```python
from build123d import *

# Parameters (mm, degrees)
F0_W     = 203.2
F0_H     = 254
F0_R     = 25.4
F1_DEPTH = 50.8
F2_R     = 5.08


with BuildPart() as f1:
    # F0 (on Top) → F1 (new body)
    with BuildSketch(Plane.XY):
        with Locations((101.6, 127)):
            Rectangle(F0_W, F0_H)
        with Locations((101.6, 50.8)):
            Circle(F0_R, mode=Mode.SUBTRACT)
        with Locations((101.6, 203.2)):
            Circle(F0_R, mode=Mode.SUBTRACT)
    extrude(amount=F1_DEPTH)

    # F2
    f2_edges = [f1.edges().sort_by_distance(p)[0] for p in [
        (101.6, 254, 0),
        (76.2, 203.2, 0),
        (0, 127, 0),
        (0, 127, 50.8),
        (0, 254, 25.4),
        (76.2, 50.8, 0),
        (203.2, 127, 0),
        (101.6, 0, 0),
        (0, 0, 25.4),
        (76.2, 203.2, 50.8),
        (76.2, 50.8, 50.8),
        (203.2, 0, 25.4),
        (101.6, 0, 50.8),
        (203.2, 127, 50.8),
    ]]
    fillet(f2_edges, radius=F2_R)


solid = f1.part
```
Read the model definition and answer for the solid it produces. Units are mm, in the model's axes. Round coordinates to 2 decimals unless told otherwise and drop trailing zeros. Loops run counter-clockwise (first coordinate to the right, second up) from the corner with the lowest first, then second, coordinate; pieces in that order, holes last. Notation, with made-up numbers: (-4, -37) -> (39, -37) arc R26 cw to (39, -2) -> close; hole circle Ø3 at (27.25, 7.25). An arc over 180 degrees is marked (long way). One line per item, written item: value.
1) The mould has two halves that part along Y. Classify faces 1 (the face through (98.293, 228.384, 25.116)), 2 (the face through (102.951, 1.449, 49.272)), 3 (the face through (201.751, 131.282, 1.528)): pulls with the +Y half, pulls with the -Y half, needs draft (parallel to the pull), parting line crosses it, or undercut.
Answer list:
face 1: undercut
face 2: pulls with the -Y half
face 3: needs draft
2) Consider L1, parallel to Y at x = 101, z = 25; L2, parallel to X at y = 203, z = 26; L3, parallel to Y at x = 103.5, z = 44.5. Determine where each line is inside the solid, lowest interval first. Write a range as [from, to].
Answer list:
L1: y = [0, 25.41], [76.19, 177.81], [228.59, 254]
L2: x = [0, 76.2], [127, 203.2]
L3: y = [0, 25.47], [76.13, 177.87], [228.53, 254]
3) A cutting plane is placed at A-A (x = 101.6). Determine the outline of the cut face in (y, z), and give its area (3 significant figures).
Answer list:
outline: (0, 5.08) arc R5.08 ccw to (5.08, 0) -> (20.32, 0) arc R5.08 ccw to (25.4, 5.08) -> (25.4, 45.72) arc R5.08 ccw to (20.32, 50.8) -> (5.08, 50.8) arc R5.08 ccw to (0, 45.72) -> close; (76.2, 5.08) arc R5.08 ccw to (81.28, 0) -> (172.72, 0) arc R5.08 ccw to (177.8, 5.08) -> (177.8, 45.72) arc R5.08 ccw to (172.72, 50.8) -> (81.28, 50.8) arc R5.08 ccw to (76.2, 45.72) -> close; (228.6, 5.08) arc R5.08 ccw to (233.68, 0) -> (248.92, 0) arc R5.08 ccw to (254, 5.08) -> (254, 50.8) -> (233.68, 50.8) arc R5.08 ccw to (228.6, 45.72) -> close
area: 7,680 mm²
4) A cutting plane is placed at B-B (y = 203.2). Determine the outline of the cut face in (x, z), and give its area (3 significant figures).
Answer list:
outline: (0, 5.08) arc R5.08 ccw to (5.08, 0) -> (71.12, 0) arc R5.08 ccw to (76.2, 5.08) -> (76.2, 45.72) arc R5.08 ccw to (71.12, 50.8) -> (5.08, 50.8) arc R5.08 ccw to (0, 45.72) -> close; (127, 5.08) arc R5.08 ccw to (132.08, 0) -> (198.12, 0) arc R5.08 ccw to (203.2, 5.08) -> (203.2, 45.72) arc R5.08 ccw to (198.12, 50.8) -> (132.08, 50.8) arc R5.08 ccw to (127, 45.72) -> close
area: 7,700 mm²
5) A cutting plane is placed at C-C (z = 19). Determine the outline of the cut face in (x, y).
Answer list:
outline: (0, 5.08) arc R5.08 ccw to (5.08, 0) -> (198.12, 0) arc R5.08 ccw to (203.2, 5.08) -> (203.2, 254) -> (5.08, 254) arc R5.08 ccw to (0, 248.92) -> close; hole circle Ø50.8 at (101.6, 50.8); hole circle Ø50.8 at (101.6, 203.2)
6) Flat-ended cylindrical pins translate along their axes: P1, Ø6, axis at x = 111, z = 8, coming from the -Y side; P2, Ø10, axis at x = 122.5, y = 63.5, coming from the +Z side. Find the tip coordinate at first contact, or state that the pin passes through.
Answer list:
P1: stops at y = 0
P2: stops at z = 50.7
